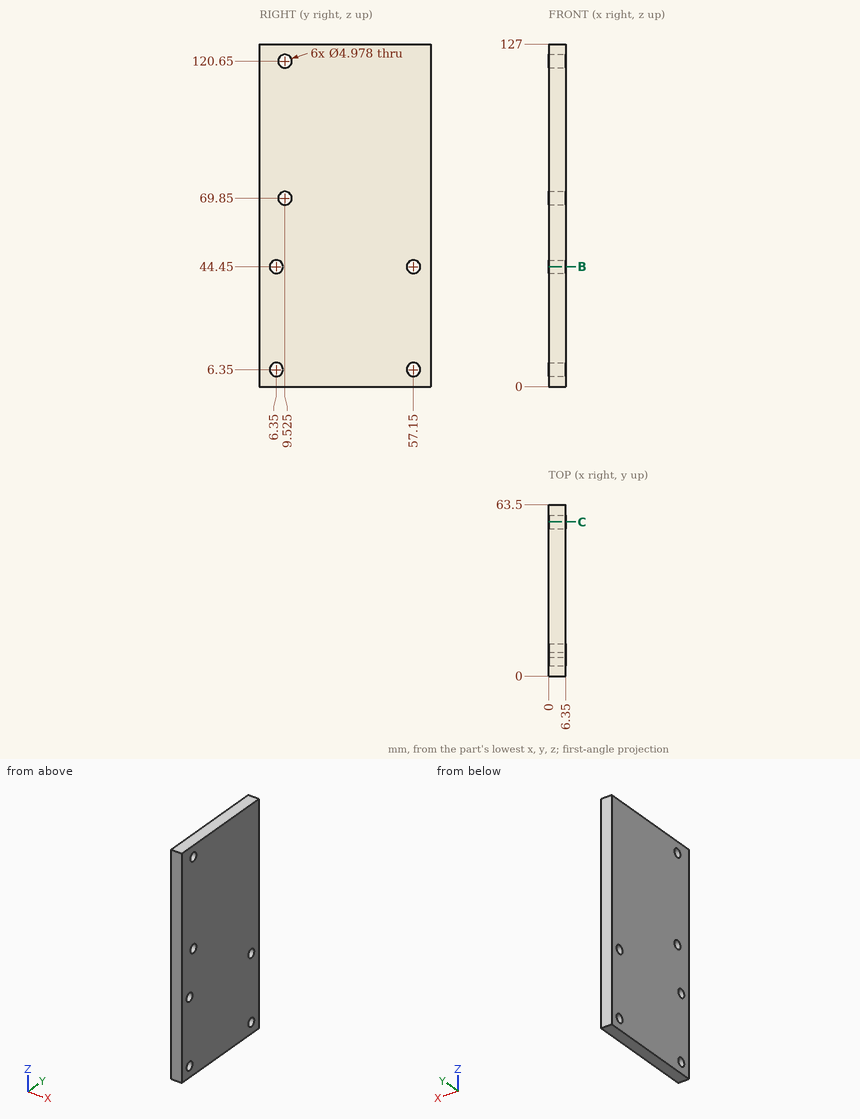
Here's the drawing with two shaded views (mm, measured from the low corner). I have some questions. Coordinates: 2 decimals unless noted, no trailing zeros. Loops run counter-clockwise (first coordinate to the right, second up) from the corner with the lowest first, then second, coordinate; pieces in that order, holes last. Notation, with made-up numbers: M 63.25,-21.5 L 97.25,-21.5 A16 ccw 97.25,8.5 Z; hole C 52.5,53.5 d5. An arc over 180 degrees is marked long. Put each result on its own line as item: value. Start each with the question number.
(1) I need wall thicknesses on probe 1 along Y at (x, z) = (3.5, 44.45); probe 2 along Y at (x, z) = (4.5, 121); probe 3 along Z at (x, y) = (0.5, 55.5) (1 decimal). Which ranges of each line are inside material? Lowest first, please.
(2) Imagine slicing it at B-B on z = 44.45. List the corners of the cut face in (x, y) for me, and give its area (3 significant figures).
(3) Imagine slicing it at C-C on y = 57.15. List the corners of the cut face in (x, z) for me.
Worked answers:
1. probe 1: y = 0 to 3.86, 8.84 to 54.66, 59.64 to 63.5
1. probe 2: y = 0 to 7.06, 11.99 to 63.5
1. probe 3: z = 0 to 4.5, 8.2 to 42.6, 46.3 to 127
2. outline: M 0,0 L 6.35,0 L 6.35,3.86 L 0,3.86 Z; M 0,8.84 L 6.35,8.84 L 6.35,54.66 L 0,54.66 Z; M 0,59.64 L 6.35,59.64 L 6.35,63.5 L 0,63.5 Z
2. area: 340 mm2
3. outline: M 0,0 L 6.35,0 L 6.35,3.86 L 0,3.86 Z; M 0,8.84 L 6.35,8.84 L 6.35,41.96 L 0,41.96 Z; M 0,46.94 L 6.35,46.94 L 6.35,127 L 0,127 Z
